For this review, take the finished solid that the model builds, in its own axes (mm). Coordinates: 2 decimals unless noted, no trailing zeros. Loops run counter-clockwise (first coordinate to the right, second up) from the corner with the lowest first, then second, coordinate; pieces in that order, holes last. Notation, with made-up numbers: M 21.5,13.5 L 35.5,13.5 A21 ccw 35.5,25.5 Z; hole C 30,42 d9. An arc over 180 degrees is marked long. Put each result on its own line as item: value.
```python
from build123d import *

# Parameters (mm, degrees)
SKETCH1_W           = 20
SKETCH1_H           = 5
SKETCH1_W_2         = 2.5
SKETCH1_H_2         = 20
BOSS_EXTRUDE1_DEPTH = 2.5


with BuildPart() as part:
    # Sketch1 → Boss-Extrude1 (new body)
    with BuildSketch(Plane.XY):
        Polygon((-72.5, 122.5), (-77.5, 122.5), (-77.5, 102.5), (-72.5, 102.5), (-72.5, 77.5), (-77.5, 77.5), (-77.5, 57.5), (-72.5, 57.5), (-72.5, 32.5), (-77.5, 32.5), (-77.5, 12.5), (-72.5, 12.5), (-72.5, -12.5), (-77.5, -12.5), (-77.5, -32.5), (-72.5, -32.5), (-72.5, -57.5), (-77.5, -57.5), (-77.5, -77.5), (-72.5, -77.5), (-72.5, -102.5), (-77.5, -102.5), (-77.5, -122.5), (-72.5, -122.5), (-72.5, -142.5), (72.5, -142.5), (72.5, -122.5), (77.5, -122.5), (77.5, -102.5), (72.5, -102.5), (72.5, -77.5), (77.5, -77.5), (77.5, -57.5), (72.5, -57.5), (72.5, -32.5), (77.5, -32.5), (77.5, -12.5), (72.5, -12.5), (72.5, 12.5), (77.5, 12.5), (77.5, 32.5), (72.5, 32.5), (72.5, 57.5), (77.5, 57.5), (77.5, 77.5), (72.5, 77.5), (72.5, 102.5), (77.5, 102.5), (77.5, 122.5), (72.5, 122.5), (72.5, 142.5), (-72.5, 142.5), align=None)
        with Locations((-47.5, 135)):
            Rectangle(SKETCH1_W, SKETCH1_H, mode=Mode.SUBTRACT)
        with Locations((-47.5, -135)):
            Rectangle(SKETCH1_W, SKETCH1_H, mode=Mode.SUBTRACT)
        with Locations((0, 135)):
            Rectangle(SKETCH1_W, SKETCH1_H, mode=Mode.SUBTRACT)
        with Locations((0, -135)):
            Rectangle(SKETCH1_W, SKETCH1_H, mode=Mode.SUBTRACT)
        with Locations((47.5, 135)):
            Rectangle(SKETCH1_W, SKETCH1_H, mode=Mode.SUBTRACT)
        with Locations((47.5, -135)):
            Rectangle(SKETCH1_W, SKETCH1_H, mode=Mode.SUBTRACT)
        with Locations((21.25, 67.5)):
            Rectangle(SKETCH1_W_2, SKETCH1_H_2, mode=Mode.SUBTRACT)
        with Locations((21.25, 112.5)):
            Rectangle(SKETCH1_W_2, SKETCH1_H_2, mode=Mode.SUBTRACT)
        with Locations((21.25, 22.5)):
            Rectangle(SKETCH1_W_2, SKETCH1_H_2, mode=Mode.SUBTRACT)
        with Locations((21.25, -22.5)):
            Rectangle(SKETCH1_W_2, SKETCH1_H_2, mode=Mode.SUBTRACT)
        with Locations((21.25, -67.5)):
            Rectangle(SKETCH1_W_2, SKETCH1_H_2, mode=Mode.SUBTRACT)
        with Locations((21.25, -112.5)):
            Rectangle(SKETCH1_W_2, SKETCH1_H_2, mode=Mode.SUBTRACT)
    extrude(amount=BOSS_EXTRUDE1_DEPTH)


solid = part.part
```
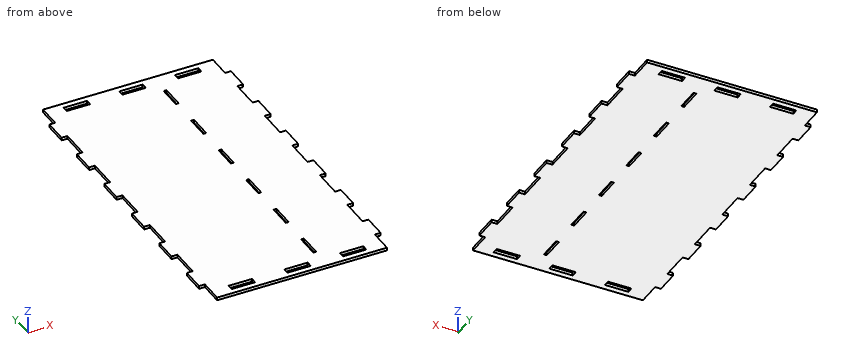
(1) Wall thickness on line 1 along Y through (x, z) = (7.5, 0.75); line 2 along X through (y, z) = (109, 2.4); line 3 along X through (y, z) = (11.5, 0.55): over which ranges is each line inside the solid? List them lowest first. Write a range as [from, to].
Determined:
line 1: y = [-142.5, -137.5], [-132.5, 132.5], [137.5, 142.5]
line 2: x = [-77.5, 20], [22.5, 77.5]
line 3: x = [-72.5, 72.5]
(2) Add section D-D (y = -45.5). Write out the cut boundary in (x, z), plus the area to 4 significant figures.
Determined:
outline: M -72.5,0 L 72.5,0 L 72.5,2.5 L -72.5,2.5 Z
area: 362.5 mm^2
(3) Add section B-B (y = 70.5). Write out the cut boundary in (x, z).
Determined:
outline: M -77.5,0 L 20,0 L 20,2.5 L -77.5,2.5 Z; M 22.5,0 L 77.5,0 L 77.5,2.5 L 22.5,2.5 Z
(4) Add section A-A (x = -41). Write out the cut boundary in (y, z), plus the area to 4 significant figures.
Determined:
outline: M -142.5,0 L -137.5,0 L -137.5,2.5 L -142.5,2.5 Z; M -132.5,0 L 132.5,0 L 132.5,2.5 L -132.5,2.5 Z; M 137.5,0 L 142.5,0 L 142.5,2.5 L 137.5,2.5 Z
area: 687.5 mm^2
(5) For pin 1 (1.2 mm diameter, centred on x = -74, z = 1, fed in from -Y), flat-tipped, find the tip position at first contact; note if it passes through.
Determined:
pin 1: stops at y = -122.5
(6) Add section C-C (z = 0.95). State how many separate pieces and enclosed holes the cut face has, plus the area to 3 significant figures.
Determined:
separate pieces: 1
enclosed holes: 12
area: 41,600 mm^2
